Here's how the part is built. I have some questions about the finished solid (model axes, mm). A direction names the side the tool comes from. Coordinates: 2 decimals unless noted, no trailing zeros. Write each loop counter-clockwise with the first axis right and the second up, starting at its lowest first coordinate (ties: lowest second). Pieces come first, ordered by that corner, then holes. Notation, with made-up numbers: (54, -26.5) -> (90, -26.5) arc R20 cw to (90, -2.5) -> close; hole circle Ø6 at (61, 43). An arc over 180 degrees is marked (long way). Use a Markdown table: item, result. Add a question column.
Item 1: Imagine slicing it at C-C, the plane z = 18.5. Write out the boundary of the cut face in (x, y).
Item 2: Imagine slicing it at A-A, the plane y = 68.5. Write out the boundary of the cut face in (x, z).
Item 3: If I drill on line 1 along Z through (x, y) = (8.5, 70); line 2 along X through (y, z) = (41, 65.5); line 3 along Y through (x, z) = (55.5, 4.5), over which ranges is the centre line in solid material (lowest first)? Write a range as from..to.
Item 4: On a 3-axis mill with a long thin cutter (end or side, diameter ignored), from which of +Z, -Z, +X, -X, +Y, -Y can I reach the whole of each face in a straight line? I mean faces 5 (the flat face through (44, 22, 35)), 6 (the flat face through (-1, 0, 40)), 7 (the cylindrical face through (0.224, 53.502, 41.209)), 8 (the flat face through (-16, 78, 31)). Say none if no direction works.
Item 5: If we mould it in two halves opening along Z, with no side actions, what happens to faces 1 (the flat face through (30, 32, 40)), 2 (the flat face through (0, 73, 50.5)), 3 (the flat face through (-1, 32, 0)), 4 (the cylindrical face through (0.224, 91.498, 40.791))? For each: pulls with the +Z half, pulls with the -Z half, needs draft (parallel to the pull), parting line crosses it, or undercut.
Item 6: Imagine slicing it at B-B, the plane y = 14. Write out the boundary of the cut face in (x, z), and give its area (3 significant figures).
Item 7: Imagine slicing it at D-D, the plane x = 27. Write out the boundary of the cut face in (y, z), and give its area (3 significant figures).
Item 8: Will these pins go through, and if not, where does the flat tip stop? pin 1 Ø8 at (x, z) = (-51.5, 29) entering from +Y; pin 2 Ø1.5 at (x, y) = (-18, 66) entering from -Z; pin 3 Ø5 at (x, y) = (5.5, 100) entering from -Z; pin 4 Ø17.5 at (x, z) = (52, 19.5) entering from +Y.
```python
from build123d import *

# Parameters (mm, degrees)
BOSS_EXTRUDE1_DEPTH = 82
CHAMFER6_SIZE       = 30
CHAMFER6_SIZE2      = 24.293520996
CHAMFER7_SIZE       = 30
CHAMFER7_SIZE2      = 24.293520996
CUT_EXTRUDE2_DEPTH  = 82


with BuildPart() as part:
    # Sketch1 → Boss-Extrude1 (new body)
    with BuildSketch(Plane.XY):
        Polygon((-60, 0), (60, 0), (60, 12), (44, 12), (44, 32), (16, 32), (16, 123), (-16, 123), (-16, 32), (-44, 32), (-44, 12), (-60, 12), align=None)
    extrude(amount=BOSS_EXTRUDE1_DEPTH)

    # Chamfer6
    chamfer6_edges = [part.edges().sort_by_distance(p)[0] for p in [
        (60, 6, 82),
    ]]
    chamfer6_side = [part.faces().sort_by_distance(p)[0] for p in [
        (60, 6, 41),
    ]]
    chamfer(chamfer6_edges, length=CHAMFER6_SIZE, length2=CHAMFER6_SIZE2, reference=chamfer6_side[0])

    # Chamfer7
    chamfer7_edges = [part.edges().sort_by_distance(p)[0] for p in [
        (-60, 6, 82),
    ]]
    chamfer7_side = [part.faces().sort_by_distance(p)[0] for p in [
        (-60, 6, 41),
    ]]
    chamfer(chamfer7_edges, length=CHAMFER7_SIZE, length2=CHAMFER7_SIZE2, reference=chamfer7_side[0])

    # Sketch8 → Cut-Extrude2 (cut)
    with BuildSketch(Plane(origin=(16, 0, 0), x_dir=(0, 0, -1), z_dir=(1, 0, 0))):
        with BuildLine():
            Line((-82, 123), (-82, 82))
            ThreePointArc((-82, 82), (-69.991378029, 110.991378029), (-41, 123))
            Line((-41, 123), (-82, 123))
        make_face()
        with BuildLine():
            ThreePointArc((-31.5, 82), (-41, 91.5), (-50.5, 82))
            Line((-50.5, 82), (-50.5, 63))
            ThreePointArc((-50.5, 63), (-41, 53.5), (-31.5, 63))
            Line((-31.5, 63), (-31.5, 82))
        make_face()
        with BuildLine():
            Line((0, 123), (-41, 123))
            ThreePointArc((-41, 123), (-12.008621971, 110.991378029), (0, 82))
            Line((0, 82), (0, 123))
        make_face()
    extrude(amount=-CUT_EXTRUDE2_DEPTH, mode=Mode.SUBTRACT)


solid = part.part
```
Ans:
| question | item | result |
|---|---|---|
| 1 | outline | (-60, 0) -> (60, 0) -> (60, 12) -> (44, 12) -> (44, 32) -> (16, 32) -> (16, 116.27) -> (-16, 116.27) -> (-16, 32) -> (-44, 32) -> (-44, 12) -> (-60, 12) -> close |
| 2 | outline | (-16, 0) -> (16, 0) -> (16, 31.5) -> (-16, 31.5) -> close; (-16, 50.5) -> (16, 50.5) -> (16, 82) -> (-16, 82) -> close |
| 3 | line 1 | z = 0..31.5, 50.5..82 |
| 3 | line 2 | x = -16..16 |
| 3 | line 3 | y = 0..12 |
| 4 | face 5 | +Z, -Z, +X, +Y |
| 4 | face 6 | +Z, -Z, +X, -X, -Y |
| 4 | face 7 | +X, -X |
| 4 | face 8 | +Z, -Z, -X, +Y |
| 5 | face 1 | needs draft |
| 5 | face 2 | undercut |
| 5 | face 3 | pulls with the -Z half |
| 5 | face 4 | undercut |
| 6 | outline | (-44, 0) -> (44, 0) -> (44, 71.76) -> (35.71, 82) -> (-35.71, 82) -> (-44, 71.76) -> close |
| 6 | area | 7,130 mm^2 |
| 7 | outline | (0, 0) -> (32, 0) -> (32, 82) -> (0, 82) -> close |
| 7 | area | 2,620 mm^2 |
| 8 | pin 1 | stops at y = 12 |
| 8 | pin 2 | passes through |
| 8 | pin 3 | stops at z = 3.04 |
| 8 | pin 4 | stops at y = 32 |
